Geometry: final body of the model. Coordinates: model frame, mm. Coordinates: 2 decimals unless noted, no trailing zeros. Order: outer loops, then holes, each group sorted by start corner. A loop starts at its lowest first (then second) coordinate and runs counter-clockwise, first axis right, second up. Notation, with made-up numbers: (79.5, 74) -> (111.5, 74) arc R11 ccw to (111.5, 91) -> close; hole circle Ø8 at (-24, 17.5). An arc over 180 degrees is marked (long way). Use CSV: the item, a comma, the result in double quotes. Start each with the question number.
from build123d import *

# Parameters (mm, degrees)
SKETCH2_R           = 6.35
BOSS_EXTRUDE1_DEPTH = 38.1


with BuildPart() as part:
    # Sketch2 → Boss-Extrude1 (new body)
    with BuildSketch(Plane.XY):
        with BuildLine():
            Line((26.443106469, -16.095077953), (63.5, -16.095077953))
            Line((63.5, -16.095077953), (63.5, -30.95625))
            Line((63.5, -30.95625), (-63.5, -30.95625))
            Line((-63.5, -30.95625), (-63.5, -16.095077953))
            Line((-63.5, -16.095077953), (-26.443106469, -16.095077953))
            ThreePointArc((-26.443106469, -16.095077953), (0, 30.95625), (26.443106469, -16.095077953))
        make_face()
        with Locations(Location((0, 0, 0), (0, 0, 180))):
            Circle(SKETCH2_R, mode=Mode.SUBTRACT)
    extrude(amount=BOSS_EXTRUDE1_DEPTH)


solid = part.part
(1) Line query: line 1 (Y direction, x = 0, z = 24.5); line 2 (Y direction, x = -31, z = 20); line 3 (X direction, y = 3, z = 3). Output: solid intervals per line, ascending. Write a range as from..to.
(2) First-contact query: pin 1 (2 mm diameter, centred on y = 16, z = 5.5, fed in from +X); pin 2 (2 mm diameter, centred on x = 12.5, z = 4, fed in from +Y); pin 3 (8 mm diameter, centred on x = 6, z = 10, fed in from +Y). Flat tips, straight axial feed; report the tip coordinate or a pass-through.
(3) Section D-D (x = -44). Return loops of the section in (y, z).
(4) Mould query, pull axis Y, two halves, no side actions, for faces 1 (the face through (0.89, -6.45, 38.1)), 2 (the face through (-0.918, 30.943, 18.783)), 3 (the face through (1, -30.956, 19)). Classes: pulls with the +Y half, pulls with the -Y half, needs draft (parallel to the pull), parting line crosses it, or undercut.
(5) Section A-A (x = 0). Return loops of the section in (y, z).
(6) Section B-B (z = 28). Return loops of the section in (x, y).
Check sheet entries:
1,line 1,"y = -30.96..-6.35, 6.35..30.96"
1,line 2,"y = -30.96..-16.1"
1,line 3,"x = -30.81..-5.6, 5.6..30.81"
2,pin 1,"stops at x = 27.08"
2,pin 2,"stops at y = 28.74"
2,pin 3,"stops at y = 30.89"
3,outline,"(-30.96, 0) -> (-16.1, 0) -> (-16.1, 38.1) -> (-30.96, 38.1) -> close"
4,face 1,"needs draft"
4,face 2,"undercut"
4,face 3,"pulls with the -Y half"
5,outline,"(-30.96, 0) -> (-6.35, 0) -> (-6.35, 38.1) -> (-30.96, 38.1) -> close; (6.35, 0) -> (30.96, 0) -> (30.96, 38.1) -> (6.35, 38.1) -> close"
6,outline,"(-63.5, -30.96) -> (63.5, -30.96) -> (63.5, -16.1) -> (26.44, -16.1) arc R30.96 ccw (long way) to (-26.44, -16.1) -> (-63.5, -16.1) -> close; hole circle Ø12.7 at (0, 0)"
